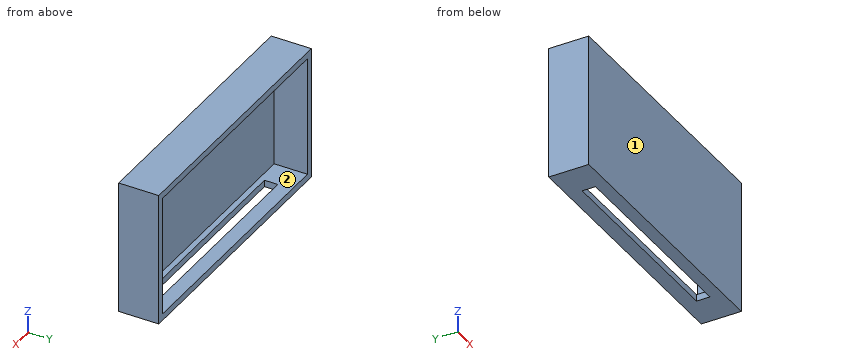
from build123d import *

# Parameters (mm, degrees)
SKETCH2_W           = 200
SKETCH2_H           = 100
BOSS_EXTRUDE1_DEPTH = 30
SHELL1_T            = -5
SKETCH3_W           = 150
SKETCH3_H           = 10
CUT_EXTRUDE1_DEPTH  = 10


with BuildPart() as part:
    # Sketch2 → Boss-Extrude1 (new body)
    with BuildSketch(Plane(origin=(0, 0, 0), x_dir=(1, 0, 0), z_dir=(0, 1, 0))):
        Rectangle(SKETCH2_W, SKETCH2_H)
    extrude(amount=BOSS_EXTRUDE1_DEPTH)

    # Shell1
    shell1_openings = [part.faces().sort_by_distance(p)[0] for p in [
        (0, 30, 0),
    ]]
    offset(amount=SHELL1_T, openings=shell1_openings, kind=Kind.INTERSECTION)

    # Sketch3 → Cut-Extrude1 (cut)
    with BuildSketch(Plane.XY.offset(-45)):
        with Locations((0, 14.223574028)):
            Rectangle(SKETCH3_W, SKETCH3_H)
    extrude(amount=-CUT_EXTRUDE1_DEPTH, mode=Mode.SUBTRACT)


solid = part.part
Part model, mm, in its own coordinate system. Face numbers are marked on the shaded views. A direction names the side the tool comes from. Round coordinates to 2 decimals unless told otherwise and drop trailing zeros. Loops run counter-clockwise (first coordinate to the right, second up) from the corner with the lowest first, then second, coordinate; pieces in that order, holes last. Notation, with made-up numbers: (80.25, -28) - (112.25, -28) arc R23 ccw to (112.25, -4) - close; hole circle Ø7 at (48.5, 72.5). An arc over 180 degrees is marked (long way). Answer as a JSON object with one key per item and string values.
Item 1: Wall check: L1, parallel to X at y = 22, z = 31.5; L2, parallel to Z at x = 12.5, y = 23; L3, parallel to Y at x = -84, z = 26.5. Give the ranges that are in metal, low to high.
Output:
{"L1": "-100 to -95, 95 to 100", "L2": "-50 to -45, 45 to 50", "L3": "0 to 5"}
Item 2: Pin check, flat tips, straight feed: pin 1 (8 mm diameter, centred on x = -32.5, z = -6.5, fed in from +Y); pin 2 (5 mm diameter, centred on x = -21, y = 12, fed in from -Z). Stop position of each tip, or through.
Output:
{"pin 1": "y = 5", "pin 2": "z = 45"}
Item 3: Band-saw the part on A-A on x = 65. List the corners of the cut face in (y, z), plus the area to 3 significant figures.
Output:
{"outline": "(0, -50) - (9.22, -50) - (9.22, -45) - (5, -45) - (5, 45) - (30, 45) - (30, 50) - (0, 50) - close; (19.22, -50) - (30, -50) - (30, -45) - (19.22, -45) - close", "area": "700 mm2"}
Item 4: Band-saw the part on B-B on z = -26.5. List the corners of the cut face in (x, y), plus the area to 3 significant figures.
Output:
{"outline": "(-100, 0) - (100, 0) - (100, 30) - (95, 30) - (95, 5) - (-95, 5) - (-95, 30) - (-100, 30) - close", "area": "1,250 mm2"}
Item 5: Tool access for the marked faces 1 and 2: list every direction of +Z, -Z, +X, -X, +Y, -Y with a clear straight run to the whole face (end or side of a thin tool).
Output:
{"face 1": "+Z, -Z, +X, -X, -Y", "face 2": "+Y"}
Item 6: Band-saw the part on C-C on y = 12.5. List the corners of the cut face in (x, z).
Output:
{"outline": "(-100, -50) - (-75, -50) - (-75, -45) - (-95, -45) - (-95, 45) - (95, 45) - (95, -45) - (75, -45) - (75, -50) - (100, -50) - (100, 50) - (-100, 50) - close"}
